Autodesk Inventor part; units mm, degrees
ref_plane "Work Plane1" through (0, 0, 0) normal (0, 0, 1) x (1, 0, 0)
ref_plane "YZ Plane" through (0, 0, 0) normal (1, 0, 0) x (0, 1, 0)
ref_plane "XZ Plane" through (0, 0, 0) normal (0, 1, 0) x (-1, 0, 0)
ref_plane "Work Plane1" through (0, 0, 0) normal (0, 0, 1) x (1, 0, 0)
sketch "Sketch1" plane through (0, 0, 0) normal (0, 0, 1) x (1, 0, 0)
  line L0 (0, 0) -> (0, 68)
  line L1 (-3.5, 0) -> (-3.5, 68)
  line L2 (0, 0) -> (-3.5, 0)
  line L3 (-3.5, 7) -> (-3.5, 0)
  line L4 (-3.5, 7) -> (-33.5, 7)
  line L5 (-33.5, 7) -> (-33.5, 0)
  line L6 (-6.5, 0) -> (-33.5, 0)
  line L7 (-3.5, 0) -> (-6.5, 0)
  line L8 (-33.5, 19) -> (-33.5, 24)
  line L9 (-33.5, 19) -> (-3.5, 19)
  line L10 (-3.5, 19) -> (-3.5, 24)
  line L11 (-3.5, 24) -> (-33.5, 24)
  line L12 (-33.5, 49) -> (-33.5, 44)
  line L13 (-3.5, 44) -> (-33.5, 44)
  line L14 (-3.5, 49) -> (-3.5, 44)
  line L15 (-33.5, 49) -> (-3.5, 49)
  line L16 (-3.5, 61) -> (-3.5, 68)
  line L17 (-3.5, 68) -> (-6.5, 68)
  line L18 (-6.5, 68) -> (-33.5, 68)
  line L19 (-33.5, 61) -> (-33.5, 68)
  line L20 (-3.5, 61) -> (-33.5, 61)
  line L21 (-34.5, 123) -> (10.5, 123)
  line L22 (10.5, -55) -> (-34.5, -55)
  line L23 (-33.5, 123) -> (-33.5, -55.3182)
  circle A0 centre (-30.5, 64.5) radius 2.3
  circle A1 centre (-11.8324, 64.5) radius 2.3
  circle A2 centre (-18.5, 21.5) radius 2.3
  circle A3 centre (-18.5, 46.5) radius 2.3
  line L24 (0, -55) -> (0, 123)
  line L25 (0, 68) -> (-3.5, 68)
  point P0 (-33.5, -55)
  dimension "d10" = 0
  dimension "d41" = 0
extrude "Extrusion1" add sketch "Sketch1" along normal blind 2 contours L2 L1 L25 L0 | L7 L6 L5 L4 L1 | L1 L20 L19 L18 L17 | L4 L23 L9 L1 | L1 L15 L23 L20 | L9 L8 L11 L1 | L1 L13 L12 L15 | L11 L23 L13 L1 | A0 | A1 | A2 | A3
sketch "Sketch2" plane through (0, 0, 2) normal (0, 0, 1) x (1, 0, 0)
  circle A0 centre (-30.5, 3.5) radius 2.3
  circle A1 centre (-11.8324, 3.5) radius 2.3
  line L0 (-3.5, 7) -> (-3.5, 0)
  line L1 (-3.5, 7) -> (-33.5, 7)
  line L2 (-33.5, 7) -> (-33.5, 0)
  line L3 (-6.5, 0) -> (-33.5, 0)
  line L4 (-3.5, 0) -> (-6.5, 0)
  circle A2 centre (-18.5, 46.5) radius 2.3
  line L5 (-33.5, 49) -> (-33.5, 44)
  line L6 (-3.5, 44) -> (-33.5, 44)
  line L7 (-3.5, 49) -> (-3.5, 44)
  line L8 (-33.5, 49) -> (-3.5, 49)
  circle A3 centre (-18.5, 21.5) radius 2.3
  line L9 (-33.5, 19) -> (-33.5, 24)
  line L10 (-33.5, 19) -> (-3.5, 19)
  line L11 (-3.5, 19) -> (-3.5, 24)
  line L12 (-3.5, 24) -> (-33.5, 24)
  circle A4 centre (-30.5, 64.5) radius 2.3
  circle A5 centre (-11.8324, 64.5) radius 2.3
  line L13 (-3.5, 61) -> (-3.5, 68)
  line L14 (-3.5, 68) -> (-6.5, 68)
  line L15 (-6.5, 68) -> (-33.5, 68)
  line L16 (-33.5, 61) -> (-33.5, 68)
  line L17 (-3.5, 61) -> (-33.5, 61)
  point P0 (0, 0)
hole "Hole1" at (-30.5, 3.5, 2) at (-11.8324, 3.5, 2) at (-18.5, 21.5, 2) at (-18.5, 46.5, 2) at (-30.5, 64.5, 2) at (-11.8324, 64.5, 2) direction (0, 0, -1) diameter 3.6 end through all countersink diameter 6 countersink angle 90
sketch "Sketch3" plane through (0, 0, 0) normal (0, 0, -1) x (-1, 0, 0)
  circle A0 centre (30.5, 3.5) radius 2.3
  circle A1 centre (11.8324, 3.5) radius 2.3
  line L0 (3.5, 7) -> (3.5, 0)
  line L1 (3.5, 7) -> (33.5, 7)
  line L2 (33.5, 7) -> (33.5, 0)
  line L3 (6.5, 0) -> (33.5, 0)
  line L4 (3.5, 0) -> (6.5, 0)
  circle A2 centre (18.5, 21.5) radius 2.3
  line L5 (33.5, 19) -> (33.5, 24)
  line L6 (33.5, 19) -> (3.5, 19)
  line L7 (3.5, 19) -> (3.5, 24)
  line L8 (3.5, 24) -> (33.5, 24)
  circle A3 centre (18.5, 46.5) radius 2.3
  line L9 (33.5, 49) -> (33.5, 44)
  line L10 (3.5, 44) -> (33.5, 44)
  line L11 (3.5, 49) -> (3.5, 44)
  line L12 (33.5, 49) -> (3.5, 49)
  circle A4 centre (30.5, 64.5) radius 2.3
  circle A5 centre (11.8324, 64.5) radius 2.3
  line L13 (3.5, 61) -> (3.5, 68)
  line L14 (3.5, 68) -> (6.5, 68)
  line L15 (6.5, 68) -> (33.5, 68)
  line L16 (33.5, 61) -> (33.5, 68)
  line L17 (3.5, 61) -> (33.5, 61)
  line L18 (33.5, 123) -> (33.5, -55)
  line L19 (33.5, 68) -> (0, 68)
  line L20 (0, 68) -> (0, 0)
  line L21 (0, 0) -> (33.5, 0)
  line L22 (33.5, 0) -> (33.5, 68)
  line L23 (31.5, 68) -> (2, 68)
  line L24 (2, 68) -> (2, 121)
  line L25 (2, 121) -> (31.5, 121)
  line L26 (31.5, 121) -> (31.5, 68)
  line L27 (31.5, 0) -> (2, 0)
  line L28 (2, 0) -> (2, -53)
  line L29 (2, -53) -> (31.5, -53)
  line L30 (31.5, -53) -> (31.5, 0)
  line L31 (0, 123) -> (33.5, 123)
  line L32 (0, -55) -> (0, 123)
  line L33 (33.5, -55) -> (0, -55)
  line L34 (2, 68) -> (31.5, 121) construction
  line L35 (31.5, 68) -> (2, 121) construction
  line L36 (31.5, 0) -> (2, -53) construction
  line L37 (31.5, -53) -> (2, 0) construction
  line L38 (3.1445, 121) -> (31.5, 70.0562)
  line L39 (2, 118.9438) -> (30.3555, 68)
  line L40 (3.1445, 68) -> (31.5, 118.9438)
  line L41 (30.3555, 121) -> (2, 70.0562)
  line L42 (3.1445, 0) -> (31.5, -50.9438)
  line L43 (30.3555, -53) -> (2, -2.0562)
  line L44 (2, -50.9438) -> (30.3555, 0)
  line L45 (31.5, -2.0562) -> (3.1445, -53)
  line L46 (31.5, 61) -> (2, 61)
  line L47 (2, 61) -> (2, 49)
  line L48 (2, 49) -> (31.5, 49)
  line L49 (31.5, 49) -> (31.5, 61)
  line L50 (31.5, 44) -> (2, 44)
  line L51 (2, 44) -> (2, 24)
  line L52 (2, 24) -> (31.5, 24)
  line L53 (31.5, 24) -> (31.5, 44)
  line L54 (31.5, 19) -> (2, 19)
  line L55 (2, 19) -> (2, 7)
  line L56 (2, 7) -> (31.5, 7)
  line L57 (31.5, 7) -> (31.5, 19)
  line L58 (31.5, 61) -> (2, 49) construction
  line L59 (31.5, 49) -> (2, 61) construction
  line L60 (2, 44) -> (31.5, 24) construction
  line L61 (31.5, 44) -> (2, 24) construction
  line L62 (2, 19) -> (31.5, 7) construction
  line L63 (31.5, 19) -> (2, 7) construction
  line L64 (2, 50.0796) -> (28.8461, 61)
  line L65 (31.5, 59.9204) -> (4.6539, 49)
  line L66 (31.5, 50.0796) -> (4.6539, 61)
  line L67 (2, 59.9204) -> (28.8461, 49)
  line L68 (29.718, 44) -> (2, 25.2082)
  line L69 (31.5, 42.7918) -> (3.782, 24)
  line L70 (2, 42.7918) -> (29.718, 24)
  line L71 (31.5, 25.2082) -> (3.782, 44)
  line L72 (31.5, 17.9204) -> (4.6539, 7)
  line L73 (2, 8.0796) -> (28.8461, 19)
  line L74 (4.6539, 19) -> (31.5, 8.0796)
  line L75 (28.8461, 7) -> (2, 17.9204)
  line L76 (33.5, 68) -> (33.5, 0)
  line L77 (33.5, 3.5) -> (33.5, 0)
  line L78 (33.5, 64.5) -> (33.5, 3.5)
  line L79 (33.5, 68) -> (33.5, 64.5)
  point P0 (16.75, -24.4438)
  point P1 (30.3555, 0)
  point P2 (3.1445, 0)
  point P3 (17.8945, -26.5)
  point P4 (16.75, -28.5562)
  point P5 (15.6055, -26.5)
  point P6 (16.75, 92.4438)
  point P7 (30.3555, 68)
  point P8 (15.6055, 94.5)
  point P9 (17.8945, 94.5)
  point P10 (16.75, 96.5562)
  point P11 (19.4039, 13)
  point P12 (28.8461, 7)
  point P13 (16.75, 11.9204)
  point P14 (4.6539, 7)
  point P15 (14.0961, 13)
  point P16 (16.75, 14.0796)
  point P17 (28.8461, 19)
  point P18 (29.718, 24)
  point P19 (16.75, 32.7918)
  point P20 (3.782, 24)
  point P21 (18.532, 34)
  point P22 (14.968, 34)
  point P23 (3.782, 44)
  point P24 (16.75, 35.2082)
  point P25 (14.0961, 55)
  point P26 (4.6539, 49)
  point P27 (16.75, 56.0796)
  point P28 (28.8461, 61)
  point P29 (19.4039, 55)
  point P30 (16.75, 53.9204)
  dimension "d11" = 2
  dimension "d12" = 2
  dimension "d13" = 2
  dimension "d14" = 2
  dimension "d15" = 2
  dimension "d16" = 2
  dimension "d17" = 1
  dimension "d18" = 1
  dimension "d19" = 1
  dimension "d20" = 1
  dimension "d21" = 1
  dimension "d22" = 1
  dimension "d23" = 1
  dimension "d24" = 1
  dimension "d27" = 2
  dimension "d28" = 2
  dimension "d29" = 1
  dimension "d30" = 1
  dimension "d31" = 1
  dimension "d32" = 1
  dimension "d33" = 1
  dimension "d34" = 1
  dimension "d35" = 1
  dimension "d36" = 1
  dimension "d37" = 1
  dimension "d38" = 1
  dimension "d39" = 1
  dimension "d40" = 1
  dimension "d42" = 0
extrude "Extrusion2" cut sketch "Sketch3" against normal blind 1 contours L4 L3 L44 L42 L21 | L72 L75 L1 | L55 L75 L73 | L72 L57 L74 | L43 L44 L28 | L45 L30 L42 | L74 L6 L73 | L43 L29 L45 | L40 L39 L15 L14 L19 | L24 L39 L41 | L69 L70 L8 | L71 L69 L53 | L51 L70 L68 | L40 L26 L38 | L38 L25 L41 | L68 L71 L10 | L17 L64 L66 | L12 L65 L67 | L66 L65 L49 | L67 L64 L47
properties part number "back" material "ABS Plastic"
Geometry check sheet. Reference: the model listing, model coordinates, mm. A direction names the side the tool comes from. Coordinates: 2 decimals unless noted, no trailing zeros. Order: outer loops, then holes, each group sorted by start corner. A loop starts at its lowest first (then second) coordinate and runs counter-clockwise, first axis right, second up. Notation, with made-up numbers: (83.5, 27.25) -> (137.5, 27.25) arc R15 ccw to (137.5, 49.25) -> close; hole circle Ø9 at (75.5, 88.25). An arc over 180 degrees is marked (long way). Use a Markdown table: item, result. Add a question column.
1. Cross-section at A-A (y = 21.5). Enter the section's corners in (x, z).
2. Cross-section at C-C (y = 37.5). Enter the section's corners in (x, z).
3. Material ranges on L1, parallel to X at y = 64.5, z = 0.2; L2, parallel to X at y = 30, z = 0.1; L3, parallel to Y at x = -30.5, z = 0.35, recorded low to high.
4. Mould release check, pull along X, two halves, no side actions. Record for faces 1 (the face through (-17, 34, 0)), 2 (the face through (-7.963, 10.505, 0.493)), 3 (the face through (0, 34, 1)): pulls with the +X half, pulls with the -X half, needs draft (parallel to the pull), parting line crosses it, or undercut.
5. Set-up check for faces 4 (the face through (-10.8, 58.5, 0.5)), 5 (the face through (-31.717, 65.827, 0.394)): record each of +Z, -Z, +X, -X, +Y, -Y from which the full face is reachable in a straight line by a thin tool's end or side.
6. Go/stop test with a flat-tipped pin: pin 1 Ø3 at (x, y) = (-28, 57) entering from -Z. Record where the tip stops, or that it passes through.
7. Cross-section at B-B (x = -30.5). Enter the section's corners in (y, z).
Filled sheet:
| question | item | result |
|---|---|---|
| 1 | outline | (-33.5, 0) -> (-20.3, 0) -> (-20.3, 0.8) -> (-21.5, 2) -> (-33.5, 2) -> close; (-16.7, 0) -> (0, 0) -> (0, 2) -> (-15.5, 2) -> (-16.7, 0.8) -> close |
| 2 | outline | (-33.5, 0) -> (-31.5, 0) -> (-31.5, 1) -> (-23.69, 1) -> (-23.69, 0) -> (-20.13, 0) -> (-20.13, 1) -> (-13.37, 1) -> (-13.37, 0) -> (-9.81, 0) -> (-9.81, 1) -> (-2, 1) -> (-2, 0) -> (0, 0) -> (0, 2) -> (-33.5, 2) -> close |
| 3 | L1 | -33.5 to -32.3, -28.7 to -13.63, -10.03 to 0 |
| 3 | L2 | -33.5 to -31.5, -24.43 to -20.87, -12.63 to -9.07, -2 to 0 |
| 3 | L3 | 0 to 1.7, 5.3 to 8.49, 17.51 to 25.89, 42.11 to 50.49, 59.51 to 62.7, 66.3 to 68 |
| 4 | face 1 | needs draft |
| 4 | face 2 | undercut |
| 4 | face 3 | pulls with the +X half |
| 5 | face 4 | -Z |
| 5 | face 5 | +Z, -Z |
| 6 | pin 1 | z = 0 |
| 7 | outline | (0, 0) -> (1.7, 0) -> (1.7, 0.8) -> (0.5, 2) -> (0, 2) -> close; (5.3, 0) -> (8.49, 0) -> (8.49, 1) -> (17.51, 1) -> (17.51, 0) -> (25.89, 0) -> (25.89, 1) -> (42.11, 1) -> (42.11, 0) -> (50.49, 0) -> (50.49, 1) -> (59.51, 1) -> (59.51, 0) -> (62.7, 0) -> (62.7, 0.8) -> (61.5, 2) -> (6.5, 2) -> (5.3, 0.8) -> close; (66.3, 0) -> (68, 0) -> (68, 2) -> (67.5, 2) -> (66.3, 0.8) -> close |
